Study the drawing (mm; zero at the part's minimum x, y, z) and answer. A direction names the side the tool comes from. Round coordinates to 2 decimals unless told otherwise and drop trailing zeros. Loops run counter-clockwise (first coordinate to the right, second up) from the corner with the lowest first, then second, coordinate; pieces in that order, holes last. Notation, with made-up numbers: (-31.5, -39) -> (-7.5, -39) arc R12 cw to (-7.5, -35) -> close; hole circle Ø11 at (13, 26). An arc over 180 degrees is marked (long way). Answer in a Markdown table with one row per item. Add a question column.
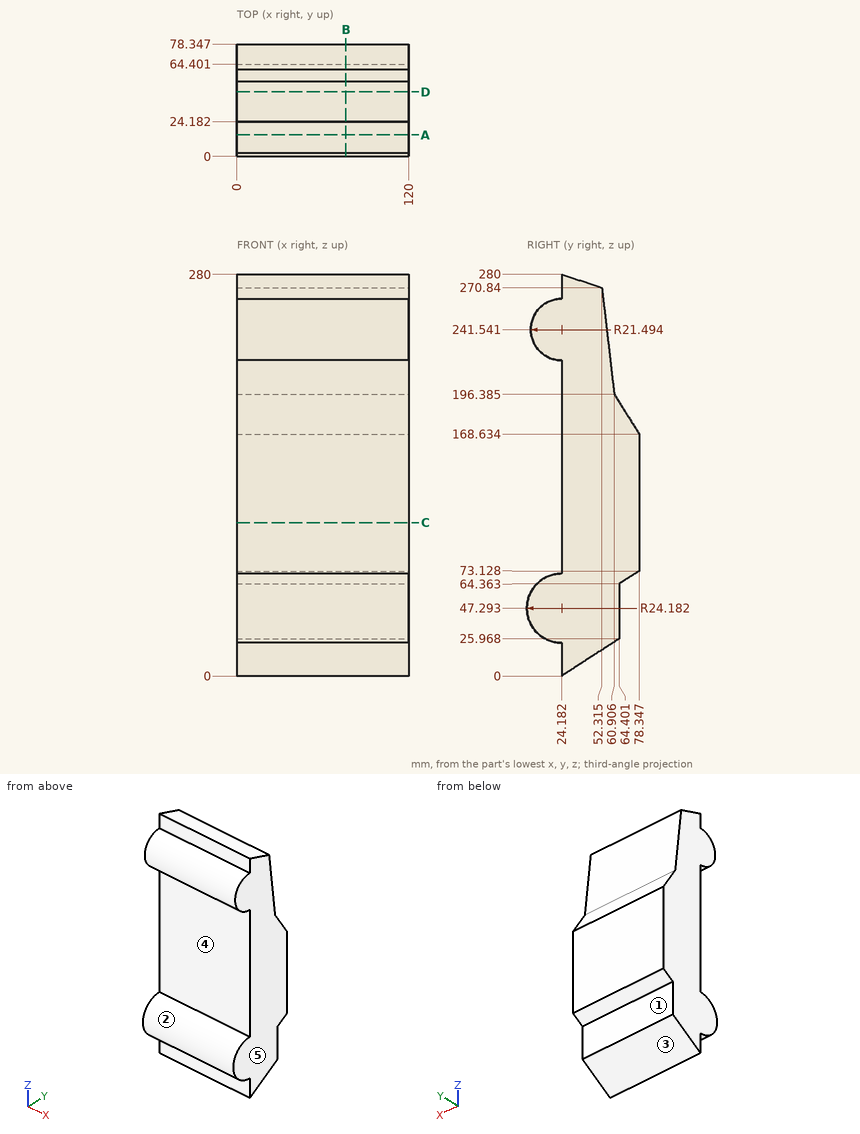
Item 1: Section A-A, the plane y = 15 is taken. Write down the section's boundary in (x, z) (1 decimal).
Item 2: For the marked faces 1 and 2, determine the directions among +Z, -Z, +X, -X, +Y, -Y from which every point of the face is accessible in a straight line to the end or side of a thin tool.
Item 3: The mould has two halves that part along Z. Classify the marked faces 3, 4 and 5: +Z half, -Z half, draft (parallel to the pull), parting line (faces both ways), or undercut.
Item 4: Section D-D, the plane y = 45 is taken. Write down the section's boundary in (x, z), and give its area (3 significant figures).
Item 5: Consider L1, parallel to Z at x = 37.5, y = 7 (1 decimal); L2, parallel to Y at x = 77.5, z = 140; L3, parallel to Z at x = 24, y = 21 (1 decimal). Determine where each line is inside the solid, lowest interval first. Write a range as from..to.
Item 6: Section C-C, the plane z = 107 is taken. Write down the section's boundary in (x, y), and give its area (3 significant figures).
Item 7: Flat-ended cylindrical pins translate along their axes: P1, Ø6, axis at x = 65, z = 109, coming from the -Y side; P2, Ø3, axis at x = 15.5, y = 66, coming from the +Z side (1 decimal); P3, Ø19, axis at x = 47.5, z = 50, coming from the +Y side. Find the tip coordinate at first contact, or state that the pin passes through.
Item 8: Section B-B, the plane x = 76 is taken. Write down the section's boundary in (y, z) (1 decimal).
Here are the results:
| question | item | result |
|---|---|---|
| 1 | outline | (0, 24.9) -> (120, 24.9) -> (120, 69.7) -> (0, 69.7) -> close; (0, 222.1) -> (120, 222.1) -> (120, 261) -> (0, 261) -> close |
| 2 | face 1 | -Z, +X, -X, +Y |
| 2 | face 2 | +X, -X, -Y |
| 3 | face 3 | -Z half |
| 3 | face 4 | undercut |
| 3 | face 5 | draft |
| 4 | outline | (0, 13.44) -> (120, 13.44) -> (120, 273.22) -> (0, 273.22) -> close |
| 4 | area | 31,200 mm² |
| 5 | L1 | z = 30.3..64.3, 228.6..254.5 |
| 5 | L2 | y = 24.18..78.35 |
| 5 | L3 | z = 23.3..71.3, 220.3..262.8 |
| 6 | outline | (0, 24.18) -> (120, 24.18) -> (120, 78.35) -> (0, 78.35) -> close |
| 6 | area | 6,500 mm² |
| 7 | P1 | stops at y = 24.18 |
| 7 | P2 | stops at z = 190.7 |
| 7 | P3 | stops at y = 64.4 |
| 8 | outline | (24.2, 0) -> (64.4, 26) -> (64.4, 64.4) -> (78.3, 73.1) -> (78.3, 168.6) -> (60.9, 196.4) -> (52.3, 270.8) -> (24.2, 280) -> (24.2, 263) arc R21.5 ccw to (24.2, 220) -> (24.2, 71.5) arc R24.2 ccw to (24.2, 23.1) -> close |
